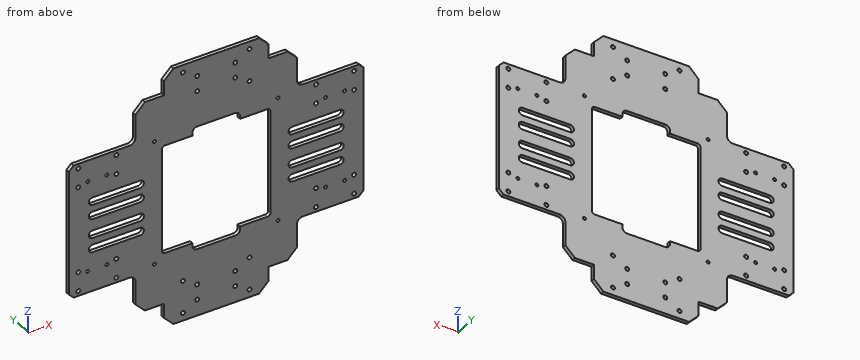
```python
from build123d import *

# Parameters (mm, degrees)
SKETCH_1_W          = 110
SKETCH_1_H          = 270.99984649
SKETCH_1_R          = 2.1
EXTRUDE_1_DEPTH     = 4
CHAMFER_1_SIZE      = 10
CUT_EXTRUDE_1_DEPTH = 4
FILLET_1_R          = 5
EXTRUDE_2_DEPTH     = 4
CHAMFER_2_SIZE      = 10
FILLET_3_R          = 5
SKETCH_5_R          = 1.6
CUT_EXTRUDE_2_DEPTH = 4
SKETCH_7_W          = 70
SKETCH_7_H          = 140
EXTRUDE_3_DEPTH     = 4
FILLET_4_R          = 6
SKETCH_8_R          = 2.1
CUT_EXTRUDE_3_DEPTH = 4
SKETCH_9_R          = 1.6
CUT_EXTRUDE_4_DEPTH = 4
CHAMFER_3_SIZE      = 5
SKETCH_11_W         = 114
SKETCH_11_H         = 114.028365308
CUT_EXTRUDE_5_DEPTH = 10
FILLET_5_R          = 3


with BuildPart() as part:
    # 草图1 → 凸台-拉伸1 (new body)
    with BuildSketch(Plane(origin=(0, 0, 0), x_dir=(1, 0, 0), z_dir=(0, 1, 0))):
        Rectangle(SKETCH_1_W, SKETCH_1_H)
        with Locations(Location((-35, 127.499923245, 0), (0, 0, 270))):
            Circle(SKETCH_1_R, mode=Mode.SUBTRACT)
        with Locations(Location((-20, 118.499923245, 0), (0, 0, 270))):
            Circle(SKETCH_1_R, mode=Mode.SUBTRACT)
        with Locations(Location((20, 118.499923245, 0), (0, 0, 270))):
            Circle(SKETCH_1_R, mode=Mode.SUBTRACT)
        with Locations(Location((35, 127.499923245, 0), (0, 0, 270))):
            Circle(SKETCH_1_R, mode=Mode.SUBTRACT)
        with Locations(Location((20, 102.499923245, 0), (0, 0, 270))):
            Circle(SKETCH_1_R, mode=Mode.SUBTRACT)
        with Locations(Location((35, 93.499923245, 0), (0, 0, 270))):
            Circle(SKETCH_1_R, mode=Mode.SUBTRACT)
        with Locations(Location((-35, 93.499923245, 0), (0, 0, 270))):
            Circle(SKETCH_1_R, mode=Mode.SUBTRACT)
        with Locations(Location((-20, 102.499923245, 0), (0, 0, 270))):
            Circle(SKETCH_1_R, mode=Mode.SUBTRACT)
        with Locations(Location((-35, -127.499923245, 0), (0, 0, 270))):
            Circle(SKETCH_1_R, mode=Mode.SUBTRACT)
        with Locations(Location((-20, -118.499923245, 0), (0, 0, 270))):
            Circle(SKETCH_1_R, mode=Mode.SUBTRACT)
        with Locations(Location((-20, -102.499923245, 0), (0, 0, 270))):
            Circle(SKETCH_1_R, mode=Mode.SUBTRACT)
        with Locations(Location((20, -118.499923245, 0), (0, 0, 270))):
            Circle(SKETCH_1_R, mode=Mode.SUBTRACT)
        with Locations(Location((20, -102.499923245, 0), (0, 0, 270))):
            Circle(SKETCH_1_R, mode=Mode.SUBTRACT)
        with Locations(Location((35, -93.499923245, 0), (0, 0, 270))):
            Circle(SKETCH_1_R, mode=Mode.SUBTRACT)
        with Locations(Location((35, -127.499923245, 0), (0, 0, 270))):
            Circle(SKETCH_1_R, mode=Mode.SUBTRACT)
    extrude(amount=EXTRUDE_1_DEPTH)

    # 倒角1
    chamfer_1_edges = [part.edges().sort_by_distance(p)[0] for p in [
        (55, 2, -135.499923245),
        (55, 2, 135.499923245),
        (-55, 2, 135.499923245),
        (-55, 2, -135.499923245),
    ]]
    chamfer(chamfer_1_edges, length=CHAMFER_1_SIZE)

    # 草图2 → 切除-拉伸1 (cut)
    with BuildSketch(Plane(origin=(0, 4, 0), x_dir=(1, 0, 0), z_dir=(0, 1, 0))):
        Polygon((-25, 45), (-40, 30), (-40, -30), (-25, -45), (-25, -65), (25, -65), (25, -45), (40, -30), (40, 30), (25, 45), (25, 65), (-25, 65), align=None)
    extrude(amount=-CUT_EXTRUDE_1_DEPTH, mode=Mode.SUBTRACT)

    # 圆角1
    fillet_1_edges = [part.edges().sort_by_distance(p)[0] for p in [
        (25, 2, -65),
        (25, 2, 65),
        (-25, 2, 65),
        (-25, 2, -65),
    ]]
    fillet(fillet_1_edges, radius=FILLET_1_R)

    # 草图3 → 凸台-拉伸2 (add)
    with BuildSketch(Plane(origin=(0, 4, 0), x_dir=(1, 0, 0), z_dir=(0, 1, 0))):
        Polygon((55, 110.499923245), (85, 110.499923245), (85, 93.499923245), (85, -102.499923245), (85, -110.499923245), (55, -110.499923245), (55, -102.499923245), (55, 93.499923245), align=None)
        Polygon((-85, 93.499923245), (-85, -102.499923245), (-85, -110.499923245), (-55, -110.499923245), (-55, -102.499923245), (-55, 93.499923245), (-55, 110.499923245), (-85, 110.499923245), align=None)
    extrude(amount=-EXTRUDE_2_DEPTH)

    # 倒角2
    chamfer_2_edges = [part.edges().sort_by_distance(p)[0] for p in [
        (-85, 2, 110.499923245),
        (85, 2, 110.499923245),
        (85, 2, -110.499923245),
        (-85, 2, -110.499923245),
    ]]
    chamfer(chamfer_2_edges, length=CHAMFER_2_SIZE)

    # 圆角3
    fillet_3_edges = [part.edges().sort_by_distance(p)[0] for p in [
        (40, 2, -30),
        (40, 2, 30),
        (-40, 2, 30),
        (-40, 2, -30),
    ]]
    fillet(fillet_3_edges, radius=FILLET_3_R)

    # 草图5 → 切除-拉伸2 (cut)
    with BuildSketch(Plane(origin=(0, 4, 0), x_dir=(1, 0, 0), z_dir=(0, 1, 0))):
        with Locations(Location((-65, 65, 0), (0, 0, 270))):
            Circle(SKETCH_5_R)
        with Locations(Location((65, 65, 0), (0, 0, 270))):
            Circle(SKETCH_5_R)
        with Locations(Location((65, -65, 0), (0, 0, 270))):
            Circle(SKETCH_5_R)
        with Locations(Location((-65, -65, 0), (0, 0, 270))):
            Circle(SKETCH_5_R)
    extrude(amount=-CUT_EXTRUDE_2_DEPTH, mode=Mode.SUBTRACT)

    # 草图7 → 凸台-拉伸3 (add)
    with BuildSketch(Plane(origin=(0, 4, 0), x_dir=(1, 0, 0), z_dir=(0, 1, 0))):
        Polygon((-85, 0), (-85, 70), (-155, 70), (-155, -70), (-85, -70), align=None)
        with Locations((120, 0)):
            Rectangle(SKETCH_7_W, SKETCH_7_H)
    extrude(amount=-EXTRUDE_3_DEPTH)

    # 圆角4
    fillet_4_edges = [part.edges().sort_by_distance(p)[0] for p in [
        (-85, 2, 70),
        (-85, 2, -70),
        (85, 2, 70),
        (85, 2, -70),
    ]]
    fillet(fillet_4_edges, radius=FILLET_4_R)

    # 草图8 → 切除-拉伸3 (cut)
    with BuildSketch(Plane(origin=(0, 4, 0), x_dir=(1, 0, 0), z_dir=(0, 1, 0))):
        with Locations(Location((105, 65, 0), (0, 0, 270))):
            Circle(SKETCH_8_R)
        with Locations(Location((145, 65, 0), (0, 0, 270))):
            Circle(SKETCH_8_R)
        with Locations(Location((145, 45, 0), (0, 0, 270))):
            Circle(SKETCH_8_R)
        with Locations(Location((105, 45, 0), (0, 0, 270))):
            Circle(SKETCH_8_R)
        with Locations(Location((145, -45, 0), (0, 0, 270))):
            Circle(SKETCH_8_R)
        with Locations(Location((145, -65, 0), (0, 0, 270))):
            Circle(SKETCH_8_R)
        with Locations(Location((105, -65, 0), (0, 0, 270))):
            Circle(SKETCH_8_R)
        with Locations(Location((105, -45, 0), (0, 0, 270))):
            Circle(SKETCH_8_R)
        with Locations(Location((-145, 65, 0), (0, 0, 270))):
            Circle(SKETCH_8_R)
        with Locations(Location((-105, 65, 0), (0, 0, 270))):
            Circle(SKETCH_8_R)
        with Locations(Location((-105, 45, 0), (0, 0, 270))):
            Circle(SKETCH_8_R)
        with Locations(Location((-145, 45, 0), (0, 0, 270))):
            Circle(SKETCH_8_R)
        with Locations(Location((-145, -45, 0), (0, 0, 270))):
            Circle(SKETCH_8_R)
        with Locations(Location((-105, -45, 0), (0, 0, 270))):
            Circle(SKETCH_8_R)
        with Locations(Location((-105, -65, 0), (0, 0, 270))):
            Circle(SKETCH_8_R)
        with Locations(Location((-145, -65, 0), (0, 0, 270))):
            Circle(SKETCH_8_R)
    extrude(amount=-CUT_EXTRUDE_3_DEPTH, mode=Mode.SUBTRACT)

    # 草图9 → 切除-拉伸4 (cut)
    with BuildSketch(Plane(origin=(0, 4, 0), x_dir=(1, 0, 0), z_dir=(0, 1, 0))):
        with Locations(Location((-135, 47.5, 0), (0, 0, 270))):
            Circle(SKETCH_9_R)
        with Locations(Location((-115, 47.5, 0), (0, 0, 90))):
            Circle(SKETCH_9_R)
        with Locations(Location((-115, -47.5, 0), (0, 0, 270))):
            Circle(SKETCH_9_R)
        with Locations(Location((-135, -47.5, 0), (0, 0, 90))):
            Circle(SKETCH_9_R)
        with Locations(Location((135, -47.5, 0), (0, 0, 270))):
            Circle(SKETCH_9_R)
        with Locations(Location((115, -47.5, 0), (0, 0, 90))):
            Circle(SKETCH_9_R)
        with Locations(Location((115, 47.5, 0), (0, 0, 270))):
            Circle(SKETCH_9_R)
        with Locations(Location((135, 47.5, 0), (0, 0, 90))):
            Circle(SKETCH_9_R)
        with BuildLine():
            Line((-130, 29.028690408), (-80, 29.028690408))
            ThreePointArc((-80, 29.028690408), (-76, 25.028690408), (-80, 21.028690408))
            Line((-80, 21.028690408), (-130, 21.028690408))
            ThreePointArc((-130, 21.028690408), (-134, 25.028690408), (-130, 29.028690408))
        make_face()
        with BuildLine():
            Line((-130, 14.028690408), (-80, 14.028690408))
            ThreePointArc((-80, 14.028690408), (-76, 10.028690408), (-80, 6.028690408))
            Line((-80, 6.028690408), (-130, 6.028690408))
            ThreePointArc((-130, 6.028690408), (-134, 10.028690408), (-130, 14.028690408))
        make_face()
        with BuildLine():
            Line((-130, -29.028690408), (-80, -29.028690408))
            ThreePointArc((-80, -29.028690408), (-76, -25.028690408), (-80, -21.028690408))
            Line((-80, -21.028690408), (-130, -21.028690408))
            ThreePointArc((-130, -21.028690408), (-134, -25.028690408), (-130, -29.028690408))
        make_face()
        with BuildLine():
            Line((-130, -14.028690408), (-80, -14.028690408))
            ThreePointArc((-80, -14.028690408), (-76, -10.028690408), (-80, -6.028690408))
            Line((-80, -6.028690408), (-130, -6.028690408))
            ThreePointArc((-130, -6.028690408), (-134, -10.028690408), (-130, -14.028690408))
        make_face()
        with BuildLine():
            Line((130, 29.028690408), (80, 29.028690408))
            ThreePointArc((80, 29.028690408), (76, 25.028690408), (80, 21.028690408))
            Line((80, 21.028690408), (130, 21.028690408))
            ThreePointArc((130, 21.028690408), (134, 25.028690408), (130, 29.028690408))
        make_face()
        with BuildLine():
            Line((130, 14.028690408), (80, 14.028690408))
            ThreePointArc((80, 14.028690408), (76, 10.028690408), (80, 6.028690408))
            Line((80, 6.028690408), (130, 6.028690408))
            ThreePointArc((130, 6.028690408), (134, 10.028690408), (130, 14.028690408))
        make_face()
        with BuildLine():
            Line((130, -29.028690408), (80, -29.028690408))
            ThreePointArc((80, -29.028690408), (76, -25.028690408), (80, -21.028690408))
            Line((80, -21.028690408), (130, -21.028690408))
            ThreePointArc((130, -21.028690408), (134, -25.028690408), (130, -29.028690408))
        make_face()
        with BuildLine():
            Line((130, -14.028690408), (80, -14.028690408))
            ThreePointArc((80, -14.028690408), (76, -10.028690408), (80, -6.028690408))
            Line((80, -6.028690408), (130, -6.028690408))
            ThreePointArc((130, -6.028690408), (134, -10.028690408), (130, -14.028690408))
        make_face()
    extrude(amount=-CUT_EXTRUDE_4_DEPTH, mode=Mode.SUBTRACT)

    # 倒角3
    chamfer_3_edges = [part.edges().sort_by_distance(p)[0] for p in [
        (155, 2, -70),
        (155, 2, 70),
        (-155, 2, 70),
        (-155, 2, -70),
    ]]
    chamfer(chamfer_3_edges, length=CHAMFER_3_SIZE)

    # 草图11 → 切除-拉伸5 (cut)
    with BuildSketch(Plane(origin=(0, 4, 0), x_dir=(1, 0, 0), z_dir=(0, 1, 0))):
        Rectangle(SKETCH_11_W, SKETCH_11_H)
    extrude(amount=-CUT_EXTRUDE_5_DEPTH, mode=Mode.SUBTRACT)

    # 圆角5
    fillet_5_edges = [part.edges().sort_by_distance(p)[0] for p in [
        (-57, 2, 57.014182654),
        (57, 2, -57.014182654),
        (57, 2, 57.014182654),
        (-57, 2, -57.014182654),
    ]]
    fillet(fillet_5_edges, radius=FILLET_5_R)


solid = part.part
```
Here's how the part is built. I have some questions about the finished solid (model axes, mm). Give positions to 0.01 mm unless a question says otherwise; leave off trailing zeros. Order: outer loops, then holes, each group sorted by start corner. A loop starts at its lowest first (then second) coordinate and runs counter-clockwise, first axis right, second up. Notation, with made-up numbers: (72, 65.25) -> (84, 65.25) arc R17 ccw to (84, 76.25) -> close; hole circle Ø2 at (45, 57). An arc over 180 degrees is marked (long way). Use CSV: the item, a comma, the result in double quotes. Start each with the question number.
Item 1: Suppose I cut it at B-B (y = 1.15). Give the number of separate pieces and of enclosed holes in the cut face, and give its area (3 significant figures).
Item 2: Suppose I cut it at A-A (z = -38.5). List the corners of the cut face in (x, y) for me.
Item 3: I'm going to push flat-ended pins straight in: P1, Ø2, axis at x = 52, y = 2.5, coming from the +Z side; P2, Ø2, axis at y = 3, z = -108, coming from the -X side; P3, Ø1.2, axis at x = -111.5, y = 1.5, coming from the -Z side. Where does each tip first touch, or does it pass through?
Item 4: If I drill on probe 1 along X at (y, z) = (2.8, 47.5); probe 2 along Z at (x, y) = (-127, 1.4); probe 3 along Z at (x, y) = (145, 2.75), over which ranges is the centre line in solid material (lowest first)? Write a range as [from, to].
Answer block:
1,separate pieces,"1"
1,enclosed holes,"52"
1,area,"44,400 mm^2"
2,outline,"(-155, 0) -> (-57, 0) -> (-57, 4) -> (-155, 4) -> close; (57, 0) -> (155, 0) -> (155, 4) -> (57, 4) -> close"
3,P1,"stops at z = 129.5"
3,P2,"stops at x = -78.5"
3,P3,"stops at z = -70"
4,probe 1,"x = [-155, -136.6], [-133.4, -116.6], [-113.4, -57], [57, 113.4], [116.6, 133.4], [136.6, 155]"
4,probe 2,"z = [-70, -29.03], [-21.03, -14.03], [-6.03, 6.03], [14.03, 21.03], [29.03, 70]"
4,probe 3,"z = [-70, -67.1], [-62.9, -47.1], [-42.9, 42.9], [47.1, 62.9], [67.1, 70]"
